Part model, mm, in its own coordinate system. A direction names the side the tool comes from. Coordinates: 2 decimals unless noted, no trailing zeros. Order: outer loops, then holes, each group sorted by start corner. A loop starts at its lowest first (then second) coordinate and runs counter-clockwise, first axis right, second up.
1) Cut at A-A (x = -29). List the corners of the cut face in (y, z).
2) Tool access for faces 4 (the cylindrical face through (-0.66, -13.689, 14.985)), 5 (the cylindrical face through (7.21, -31.87, -22.89)), 6 (the cylindrical face through (21, -30, 28)): list every direction of +Z, -Z, +X, -X, +Y, -Y with a clear straight run to the whole face (end or side of a thin tool).
3) Pin check, flat tips, straight feed: pin 1 Ø10 at (x, z) = (22.5, 8.5) entering from +Y; pin 2 Ø3 at (x, z) = (-29, 0) entering from -Y; pin 3 Ø4 at (x, y) = (2.5, -16) entering from +Z; pin 4 Ø8 at (y, z) = (-22, -0.5) entering from -X. Stop position of each tip, or through.
4) Cut at B-B (y = -43). List the corners of the cut face in (x, z), and give its area (3 significant figures).
5) Cut at D-D (z = 29.5). List the corners of the cut face in (x, y).
6) Wall check: L1, parallel to Z at x = -14.5, y = -28.5; L2, parallel to Z at x = 14, y = -30; L3, parallel to Y at x = -27, z = -15. Give the ranges that are in metal, low to high.
7) Mould opens along X. For faces 1 (the cylindrical face through (-31.38, -30.22, 0.1)), 2 (the flat face through (7, -27, 15)), 3 (the conical face through (5.44, -49.777, 1.208)) say: +X half, -X half, draft (parallel to the pull), parting line (faces both ways), or undercut.
8) Cut at C-C (z = 17). List the corners of the cut face in (x, y), and give its area (3 significant figures).
```python
from build123d import *

# Parameters (mm, degrees)
SKETCH5_R                      = 24
SKETCH5_R_2                    = 21
CUT_EXTRUDE1_DEPTH             = 3
F_3_16_0_1875_DIAMETER_HOLE1_D = 4.7625
CIRPATTERN1_COUNT              = 6


with BuildPart() as part:
    # Sketch1 → Revolve1 (revolve)
    with BuildSketch(Plane.XY, mode=Mode.PRIVATE) as revolve1_sk:
        with BuildLine():
            Line((0, 0), (-15, 0))
            Line((-15, 0), (-15, -27))
            Line((-15, -27), (-35, -27))
            Line((-35, -27), (-35, -33.35))
            Line((-35, -33.35), (-12.5, -33.35))
            Line((-12.5, -33.35), (-10, -35.85))
            Line((-10, -35.85), (-10, -45.35))
            Line((-10, -45.35), (-5.3467, -50.0033))
            Line((-5.3467, -50.0033), (-5.3467, -77.5033))
            ThreePointArc((-5.3467, -77.5033), (-4.614466953, -79.271066953), (-2.8467, -80.0033))
            Line((-2.8467, -80.0033), (0, -80.0033))
            Line((0, -80.0033), (0, 0))
        make_face()
    revolve(revolve1_sk.sketch.rotate(Axis((0, -80.0033, 0), (0, 1, 0)), 270), axis=Axis((0, -80.0033, 0), (0, 1, 0)))

    # Sketch4 → 1/16 NPT Tapped Hole1 (revolve, cut)
    with BuildSketch(Plane(origin=(0, 0, 0), x_dir=(0, 0, 1), z_dir=(1, 0, 0))):
        Polygon((0, 0), (0, 78.846685027), (3.0734, 77), (3.0734, 6.89), (3.829121997, 6.89), (3.968877, 2.222373), (6.19125, 0), align=None)
    revolve(axis=Axis((0, 6.35, 0), (0, -1, 0)), mode=Mode.SUBTRACT)

    # Sketch5 → Cut-Extrude1 (cut)
    with BuildSketch(Plane(origin=(0, -33.35, 0), x_dir=(-1, 0, 0), z_dir=(0, -1, 0))):
        with Locations(Location((0, 0, 0), (0, 0, 90))):
            Circle(SKETCH5_R)
        with Locations(Location((0, 0, 0), (0, 0, 90))):
            Circle(SKETCH5_R_2, mode=Mode.SUBTRACT)
    extrude(amount=-CUT_EXTRUDE1_DEPTH, mode=Mode.SUBTRACT)

    # 3/16 (0.1875) Diameter Hole1 (through all)
    with Locations(Plane(origin=(0, -27, 0), x_dir=(1, 0, 0), z_dir=(0, 1, 0))):
        with Locations((29, 0)):
            f_3_16_0_1875_diameter_hole1 = Hole(F_3_16_0_1875_DIAMETER_HOLE1_D / 2)

    # CirPattern1: 3/16 (0.1875) Diameter Hole1 ×6 about axis
    cirpattern1_axis = Axis((0, 0, 0), (0, 1, 0))
    for i in range(1, CIRPATTERN1_COUNT):
        add(f_3_16_0_1875_diameter_hole1.rotate(cirpattern1_axis, i * 360 / CIRPATTERN1_COUNT), mode=Mode.SUBTRACT)


solid = part.part
```
Geometry check:
1. outline: (-33.35, -19.6) - (-27, -19.6) - (-27, -2.38) - (-33.35, -2.38) - close; (-33.35, 2.38) - (-27, 2.38) - (-27, 19.6) - (-33.35, 19.6) - close
2. face 4: +Y
2. face 5: -Y
2. face 6: +Y, -Y
3. pin 1: stops at y = -27
3. pin 2: passes through
3. pin 3: stops at z = 14.99
3. pin 4: stops at x = -15
4. outline: circle Ø20 at (0, 0); hole circle Ø6.15 at (0, 0)
4. area: 284 mm2
5. outline: (-18.83, -33.35) - (18.83, -33.35) - (18.83, -27) - (-18.83, -27) - close
6. L1: z = -31.86 to -27.5, -22.73 to 22.73, 27.5 to 31.86
6. L2: z = -32.08 to -27.44, -22.79 to 22.79, 27.44 to 32.08
6. L3: y = -33.35 to -27
7. face 1: undercut
7. face 2: draft
7. face 3: parting line
8. outline: (-30.59, -33.35) - (-16.94, -33.35) - (-16.94, -30.35) - (-12.33, -30.35) - (-12.33, -33.35) - (12.33, -33.35) - (12.33, -30.35) - (16.94, -30.35) - (16.94, -33.35) - (30.59, -33.35) - (30.59, -27) - (-30.59, -27) - close
8. area: 361 mm2
